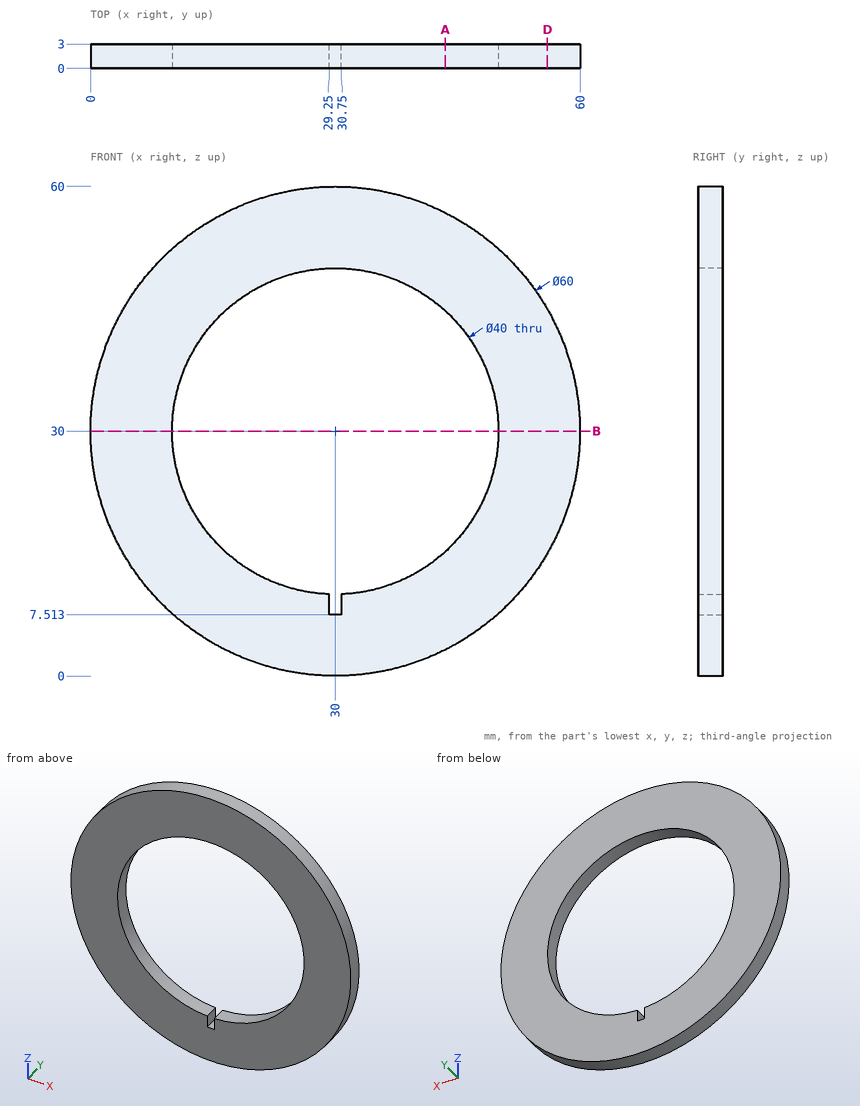
Geometry: see drawing. Coordinates: mm, zero at the bounding-box minimum. Round coordinates to 2 decimals unless told otherwise and drop trailing zeros. Order: outer loops, then holes, each group sorted by start corner. A loop starts at its lowest first (then second) coordinate and runs counter-clockwise, first axis right, second up. Notation, with made-up numbers: (70.5, 11) - (94.5, 11) arc R25 ccw to (94.5, 34) - close; hole circle Ø2 at (68.25, 17.25). An arc over 180 degrees is marked (long way). One line per question, with ' | ' between items. Start each with the question number.
1) Ray query, probe 1 along X at (y, z) = (1.8, 30); probe 2 along Z at (x, y) = (40, 2.15) (1 decimal); probe 3 along X at (y, z) = (1.25, 39). Return the intervals inside material, ascending.
2) Cut plane B-B, the plane z = 30. Return the cut outline in (x, y).
3) Contact query for flat-ended pins moving along their axis: P1, Ø1, axis at x = 37, z = 13, coming from the -Y side; P2, Ø1.5, axis at y = 2, z = 49, coming from the -X side; P3, Ø0.8, axis at y = 2, z = 9, coming from the +X side. Output: stop coordinate, or through.
4) Cut plane D-D, the plane x = 56. Return the cut outline in (y, z).
5) Cut plane A-A, the plane x = 43.5. Return the cut outline in (y, z).
Worked out:
1) probe 1: x = 0 to 10, 50 to 60 | probe 2: z = 1.7 to 12.7, 47.3 to 58.3 | probe 3: x = 1.38 to 12.14, 47.86 to 58.62
2) outline: (0, 0) - (10, 0) - (10, 3) - (0, 3) - close; (50, 0) - (60, 0) - (60, 3) - (50, 3) - close
3) P1: passes through | P2: stops at x = 6.19 | P3: stops at x = 51.81
4) outline: (0, 15.03) - (3, 15.03) - (3, 44.97) - (0, 44.97) - close
5) outline: (0, 3.21) - (3, 3.21) - (3, 15.24) - (0, 15.24) - close; (0, 44.76) - (3, 44.76) - (3, 56.79) - (0, 56.79) - close
